```python
from build123d import *

# Parameters (mm, degrees)
SKETCH1_R           = 1.5
BOSS_EXTRUDE5_DEPTH = 2


with BuildPart() as part:
    # Sketch1 → Boss-Extrude5 (new body)
    with BuildSketch(Plane.XY):
        with BuildLine():
            Line((-96.208405317, 32.365381328), (-96.208405317, 3.615381328))
            Line((-96.208405317, 3.615381328), (-78.208405317, 3.615381328))
            Line((-78.208405317, 3.615381328), (-78.208405317, -7.634618672))
            Line((-78.208405317, -7.634618672), (-78.208405317, -18.884618672))
            Line((-78.208405317, -18.884618672), (-96.208405317, -18.884618672))
            Line((-96.208405317, -18.884618672), (-96.208405317, -47.634618672))
            ThreePointArc((-96.208405317, -47.634618672), (-93.279473129, -54.705686484), (-86.208405317, -57.634618672))
            Line((-86.208405317, -57.634618672), (93.786822591, -57.634618672))
            ThreePointArc((93.786822591, -57.634618672), (100.857890403, -54.705686484), (103.786822591, -47.634618672))
            Line((103.786822591, -47.634618672), (103.786822591, -18.884618672))
            Line((103.786822591, -18.884618672), (85.791594683, -18.884618672))
            Line((85.791594683, -18.884618672), (85.791594683, -7.634618672))
            Line((85.791594683, -7.634618672), (85.791594683, 3.615381328))
            Line((85.791594683, 3.615381328), (103.786822591, 3.615381328))
            Line((103.786822591, 3.615381328), (103.786822591, 32.365381328))
            ThreePointArc((103.786822591, 32.365381328), (100.857890403, 39.43644914), (93.786822591, 42.365381328))
            add(Edge.make_bspline(
                [(93.786822591, 42.365381328), (80.365609536, 42.377038483), (3.810151403, -1.044125651), (-72.829077796, 42.354133189), (-86.208405317, 42.365381328)],
                knots=[0, 0, 0, 0, 0.5, 1, 1, 1, 1], degree=3))
            ThreePointArc((-86.208405317, 42.365381328), (-93.279473129, 39.43644914), (-96.208405317, 32.365381328))
        make_face()
        with Locations((93.786822591, 32.365381328)):
            Circle(SKETCH1_R, mode=Mode.SUBTRACT)
        with Locations((-86.208405317, 32.365381328)):
            Circle(SKETCH1_R, mode=Mode.SUBTRACT)
        with Locations((-86.208405317, -47.634618672)):
            Circle(SKETCH1_R, mode=Mode.SUBTRACT)
        with Locations((101.306428837, 6.128192253)):
            Circle(SKETCH1_R, mode=Mode.SUBTRACT)
        with Locations((83.303914286, 6.128192253)):
            Circle(SKETCH1_R, mode=Mode.SUBTRACT)
        with Locations((83.103049409, -21.36518771)):
            Circle(SKETCH1_R, mode=Mode.SUBTRACT)
        with Locations((101.306428837, -21.498180437)):
            Circle(SKETCH1_R, mode=Mode.SUBTRACT)
        with Locations((-93.738164493, 6.128192253)):
            Circle(SKETCH1_R, mode=Mode.SUBTRACT)
        with Locations((-75.737858718, 6.128192253)):
            Circle(SKETCH1_R, mode=Mode.SUBTRACT)
        with Locations((-75.737858718, -21.36518771)):
            Circle(SKETCH1_R, mode=Mode.SUBTRACT)
        with Locations((-93.738164493, -21.36518771)):
            Circle(SKETCH1_R, mode=Mode.SUBTRACT)
        with Locations((93.786822591, -47.634618672)):
            Circle(SKETCH1_R, mode=Mode.SUBTRACT)
    extrude(amount=BOSS_EXTRUDE5_DEPTH)


solid = part.part
```
Here's how the part is built. I have some questions about the finished solid (model axes, mm). Coordinates: 2 decimals unless noted, no trailing zeros. Write each loop counter-clockwise with the first axis right and the second up, starting at its lowest first coordinate (ties: lowest second). Pieces come first, ordered by that corner, then holes. Notation, with made-up numbers: (51.25, -37) - (79.25, -37) arc R15 ccw to (79.25, -23) - close; hole circle Ø10 at (29.25, 56.5). An arc over 180 degrees is marked (long way). One line per item, written item: value.
1) I need wall thicknesses on line 1 along Y through (x, z) = (-86, 0.6); line 2 along Y through (x, z) = (-87, 1.7); line 3 along X through (y, z) = (6.5, 1.55). Which ranges of each line are inside material? Lowest first, please.
Model answer:
line 1: y = -57.63 to -49.12, -46.15 to -18.88, 3.62 to 30.88, 33.85 to 42.36
line 2: y = -57.6 to -48.91, -46.36 to -18.88, 3.62 to 31.09, 33.64 to 42.33
line 3: x = -96.21 to -95.19, -92.28 to -77.19, -74.28 to 81.85, 84.76 to 99.85, 102.76 to 103.79
2) Suppose I cut it at B-B on z = 1. State how many separate pieces and enclosed holes the cut face has, and give its area (3 significant figures).
Model answer:
separate pieces: 1
enclosed holes: 12
area: 16,700 mm²
3) I'm going to push flat-ended pins straight in: P1, Ø2.5, axis at x = -93.74, y = 6.13, coming from the +Z side; P2, Ø1, axis at y = -12.5, z = 1.5, coming from the -X side; P3, Ø0.6, axis at x = -87.5, z = 1, coming from the -Y side; P4, Ø1, axis at y = -3, z = 0.5, coming from the +X side. Where does each tip first touch, or does it pass through?
Model answer:
P1: passes through
P2: stops at x = -78.21
P3: stops at y = -57.59
P4: stops at x = 85.79
4) Suppose I cut it at A-A on y = -11.5. Write out the boundary of the cut face in (x, z).
Model answer:
outline: (-78.21, 0) - (85.79, 0) - (85.79, 2) - (-78.21, 2) - close
